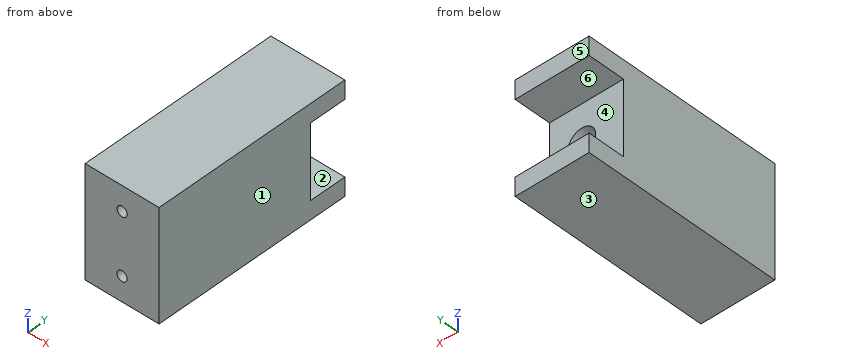
Autodesk Inventor part; units mm, degrees
ref_plane "YZ Plane" through (0, 0, 0) normal (1, 0, 0) x (0, 1, 0)
ref_plane "XZ Plane" through (0, 0, 0) normal (0, 1, 0) x (-1, 0, 0)
ref_plane "XY Plane" through (0, 0, 0) normal (0, 0, 1) x (1, 0, 0)
sketch "Sketch1" plane through (0, 0, 0) normal (0, 1, 0) x (-1, 0, 0)
  line L0 (0, 0) -> (25.4, 0)
  line L1 (25.4, 0) -> (25.4, -38.1)
  line L2 (25.4, -38.1) -> (0, -38.1)
  line L3 (0, -38.1) -> (0, 0)
  dimension "d0" = 38.1
  dimension "d1" = 25.4
extrude "Extrusion1" add sketch "Sketch1" along normal blind 68.58
sketch "Sketch2" plane through (0, 68.58, 0) normal (0, 1, 0) x (1, 0, 0)
  line L0 (0, 0) -> (0, 38.1)
  line L1 (-25.4, 38.1) -> (-25.4, 0)
  line L2 (0, 6.35) -> (-25.4, 6.35)
  line L3 (-25.4, 6.35) -> (-25.4, 31.75)
  line L4 (-25.4, 31.75) -> (0, 31.75)
  line L5 (0, 31.75) -> (0, 6.35)
  line L6 (-25.4, 0) -> (0, 0)
  dimension "d4" = 6.35
  dimension "d5" = 25.4
extrude "Extrusion2" cut sketch "Sketch2" against normal blind 12.7 contours L2 L1 L4 L0
sketch "Sketch3" plane through (0, 55.88, 0) normal (0, 1, 0) x (1, 0, 0)
  circle A0 centre (-11.1125, 19.05) radius 6.35
  point P0 (0, 0)
hole "Hole1" at (-11.1125, 55.88, -19.05) direction (0, -1, 0) diameter 9.525 depth 6.35 tip angle 118
sketch "Sketch4" plane through (0, 0, 0) normal (0, -1, 0) x (1, 0, 0)
  circle A0 centre (-11.1125, -19.05) radius 4.7625
  line L0 (-25.4, 0) -> (-25.4, -38.1)
  line L1 (0, -38.1) -> (0, 0)
  line L2 (-25.4, -38.1) -> (0, -38.1)
  line L3 (0, 0) -> (-25.4, 0)
  point P0 (-12.7, -29.6333)
  point P1 (-12.7, -8.4667)
  dimension "d15" = 25.4
  dimension "d16" = 12.7
  dimension "d17" = 12.7
  dimension "d18" = 8.4667
  dimension "d19" = 8.4667
hole "Hole2" at (-12.7, 0, -29.6333) at (-12.7, 0, -8.4667) direction (0, 1, 0) diameter 3.5052 depth 6.35 tip angle 118
properties part number "TSV+Support"
Geometry: final body of the model. Coordinates: model frame, mm. Face numbers are marked on the shaded views. A direction names the side the tool comes from. Round coordinates to 2 decimals unless told otherwise and drop trailing zeros. Loops run counter-clockwise (first coordinate to the right, second up) from the corner with the lowest first, then second, coordinate; pieces in that order, holes last. Notation, with made-up numbers: M 65.25,-27 L 90.25,-27 A20 ccw 90.25,-11 Z; hole C -25,10 d8. An arc over 180 degrees is marked long. Put each result on its own line as item: value. Start each with the question number.
(1) Draft query along Z for the marked faces 1, 2, 3 and 4. Return one class per face: +Z half, -Z half, draft (parallel to the pull), parting line (faces both ways), or undercut.
(2) Set-up query: the marked faces 5 and 6. Return all of +Z, -Z, +X, -X, +Y, -Y with unobstructed straight access to the full face (end or side cutting, diameter ignored); none if empty.
(3) Section query A-A (x = -2.75). Return loops of the section in (y, z).
(4) Contact query for flat-ended pins moving along their axis: pin 1 Ø8 at (x, z) = (-15.5, -13) entering from +Y; pin 2 Ø5.5 at (x, z) = (-11.11, -19.05) entering from +Y; pin 3 Ø3 at (x, z) = (-12.7, -8.47) entering from -Y. Output: stop coordinate, or through.
(5) Material intervals for line 1 along Z through (x, y) = (-12.7, 2.5); line 2 along Z through (x, y) = (-15.5, 60); line 3 along Y through (x, z) = (-16, -10.5), sorted ascending. Write a range as [from, to].
Findings below:
1. face 1: draft
1. face 2: undercut
1. face 3: -Z half
1. face 4: undercut
2. face 5: +Z, -Z, +X, -X, +Y
2. face 6: +X, -X, +Y
3. outline: M 0,-38.1 L 68.58,-38.1 L 68.58,-31.75 L 55.88,-31.75 L 55.88,-6.35 L 68.58,-6.35 L 68.58,0 L 0,0 Z
4. pin 1: stops at y = 55.88
4. pin 2: stops at y = 48.32
4. pin 3: stops at y = 6.5
5. line 1: z = [-38.1, -31.39], [-27.88, -10.22], [-6.71, 0]
5. line 2: z = [-38.1, -31.75], [-6.35, 0]
5. line 3: y = [0, 55.88]
